For this review, take the finished solid that the model builds, in its own axes (mm). Face numbers are marked on the shaded views. A direction names the side the tool comes from. Coordinates: 2 decimals unless noted, no trailing zeros. Order: outer loops, then holes, each group sorted by start corner. A loop starts at its lowest first (then second) coordinate and runs counter-clockwise, first axis right, second up. Notation, with made-up numbers: (59.5, 19.25) -> (77.5, 19.25) arc R23 cw to (77.5, 35.25) -> close; hole circle Ø9 at (0.25, 58.25). An arc over 180 degrees is marked (long way). Answer as a JSON object with one key per item and string values. Group by question number.
1) Add section A-A, the plane y = -1. Count the separate pieces of the cut face and the enclosed holes in it, then the cut area to 3 significant figures.
2) Add section D-D, the plane y = 27. Write out the cut boundary in (x, z).
3) Machinability: for the marked faces 1, 2 and 3, which of the approach directions +Z, -Z, +X, -X, +Y, -Y give a long, thin tool a straight path to every point of the face, cutting with its end or side? Answer none if there is none.
4) Add section C-C, the plane x = 15.5. Write out the cut boundary in (y, z), then the cut area to 3 significant figures.
5) Draft analysis for pull direction Y (two halves, no side actions). For the marked faces 4, 5 and 6, state which applies: +Y half, -Y half, draft (parallel to the pull), parting line (faces both ways), or undercut.
6) For pin 1 (6 mm diameter, centred on x = -12.5, y = 18, fed in from -Z); pin 2 (5 mm diameter, centred on y = 16.5, z = 11, fed in from +X); pin 3 (3.5 mm diameter, centred on x = 7.5, y = 28.42, fed in from -Z); pin 4 (17.5 mm diameter, centred on x = -35, y = -1, fed in from +Z), all flat-tipped, find the tip position at first contact; note any pin that passes through.
7) Add section B-B, the plane x = -17.5. Write out the cut boundary in (y, z).
8) Wall thickness on L1, parallel to Y at x = 7.5, z = 14.1; L2, parallel to X at y = 0, z = 12.75; L3, parallel to Y at x = -9, z = 5.75: over which ranges is each line inside the solid? List them lowest first.
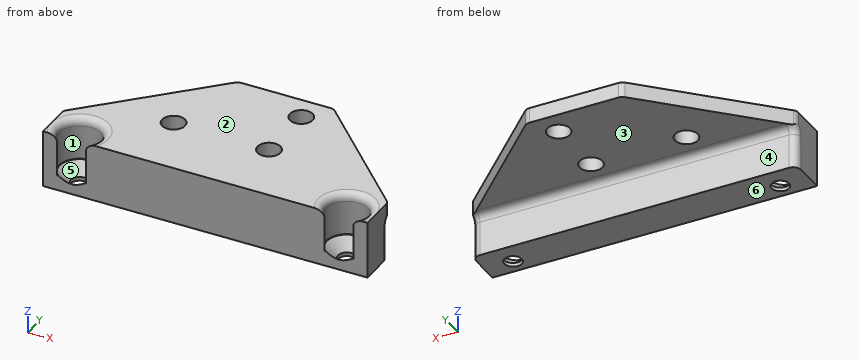
from build123d import *

# Parameters (mm, degrees)
SKETCH1_W           = 85
SKETCH1_H           = 10
BOSS_EXTRUDE1_DEPTH = 15
SKETCH3_R           = 2.292918
CUT_EXTRUDE1_DEPTH  = 100
LPATTERN1_COUNT     = 2
LPATTERN1_PITCH     = 70
SKETCH7_W           = 85
SKETCH7_H           = 4
BOSS_EXTRUDE5_DEPTH = 30
SKETCH8_R           = 3
CUT_EXTRUDE2_DEPTH  = 25
LPATTERN2_START     = 11
LPATTERN2_OUTLINE_R = 3
LPATTERN2_DEPTH     = 4
CHAMFER2_SIZE       = 30
FILLET3_START       = -1
FILLET3_DEPTH       = 10
FILLET3_START_2     = 1.5411
FILLET3_2_DEPTH     = 14.4589
FILLET3_START_3     = 9
FILLET3_3_DEPTH     = 2.164784
FILLET3_5_DEPTH     = 2
FILLET3_START_4     = 11
FILLET3_6_OUTLINE_R = 3
FILLET3_6_DEPTH     = 0.164784
SKETCH9_R           = 5.5
CUT_EXTRUDE7_DEPTH  = 11
LPATTERN3_COUNT     = 2
LPATTERN3_PITCH     = 70
CHAMFER3_SIZE       = 3
FILLET4_R           = 2


with BuildPart() as part:
    # Sketch1 → Boss-Extrude1 (new body)
    with BuildSketch(Plane.XY):
        Rectangle(SKETCH1_W, SKETCH1_H)
    extrude(amount=BOSS_EXTRUDE1_DEPTH)

    # Sketch3 → Cut-Extrude1 (cut)
    with BuildSketch(Plane.XY.offset(15)):
        with Locations((-35, -1)):
            Circle(SKETCH3_R)
    cut_extrude1 = extrude(amount=-CUT_EXTRUDE1_DEPTH, mode=Mode.SUBTRACT)

    # LPattern1: Cut-Extrude1 ×2
    with Locations(*[(i * LPATTERN1_PITCH, 0, 0) for i in range(1, LPATTERN1_COUNT)]):
        add(cut_extrude1, mode=Mode.SUBTRACT)

    # Sketch7 → Boss-Extrude5 (add)
    with BuildSketch(Plane(origin=(0, 5, 0), x_dir=(1, 0, 0), z_dir=(0, 1, 0))):
        with Locations((0, -13)):
            Rectangle(SKETCH7_W, SKETCH7_H)
    extrude(amount=BOSS_EXTRUDE5_DEPTH)

    # Sketch8 → Cut-Extrude2 (cut)
    with BuildSketch(Plane.XY.offset(15)):
        with Locations((7.5, 12.421962)):
            Circle(SKETCH8_R)
    extrude(amount=-CUT_EXTRUDE2_DEPTH, mode=Mode.SUBTRACT)

    # LPattern2: read off the stored shape, not the designer's step
    # LPattern2 outline → LPattern2 (cut)
    with BuildSketch(Plane.XY.offset(LPATTERN2_START)):
        with Locations((-17.5, 12.421962)):
            Circle(LPATTERN2_OUTLINE_R)
        with Locations((7.5, 28.421962)):
            Circle(LPATTERN2_OUTLINE_R)
    extrude(amount=LPATTERN2_DEPTH, mode=Mode.SUBTRACT)

    # Chamfer2
    chamfer2_edges = [part.edges().sort_by_distance(p)[0] for p in [
        (42.5, 35, 13),
        (-42.5, 35, 13),
    ]]
    chamfer(chamfer2_edges, length=CHAMFER2_SIZE)

    # Fillet3: read off the stored shape, not the designer's step
    # Fillet3 outline → Fillet3 (cut)
    with BuildSketch(Plane.XY.offset(FILLET3_START)):
        with BuildLine():
            ThreePointArc((40.5, 5), (41.914214, 4.414214), (42.5, 3))
            Line((42.5, 3), (42.5, 5))
            Line((42.5, 5), (40.5, 5))
        make_face()
        with BuildLine():
            ThreePointArc((-42.5, 3), (-41.914214, 4.414214), (-40.5, 5))
            Line((-40.5, 5), (-42.5, 5))
            Line((-42.5, 5), (-42.5, 3))
        make_face()
    extrude(amount=FILLET3_DEPTH, mode=Mode.SUBTRACT)

    # Fillet3 2 outline → Fillet3 2 (cut)
    with BuildSketch(Plane.XY.offset(FILLET3_START_2)):
        with BuildLine():
            Line((42.5, 4.171573), (42.5, 5))
            Line((42.5, 5), (41.914214, 5.585786))
            ThreePointArc((41.914214, 5.585786), (42.347759, 4.93694), (42.5, 4.171573))
        make_face()
        with BuildLine():
            Line((-41.914214, 5.585786), (-42.5, 5))
            Line((-42.5, 5), (-42.5, 4.171573))
            ThreePointArc((-42.5, 4.171573), (-42.347759, 4.93694), (-41.914214, 5.585786))
        make_face()
        with BuildLine():
            ThreePointArc((11.671573, 35), (12.43694, 34.847759), (13.085786, 34.414214))
            Line((13.085786, 34.414214), (12.5, 35))
            Line((12.5, 35), (11.671573, 35))
        make_face()
        with BuildLine():
            Line((-12.5, 35), (-13.085786, 34.414214))
            ThreePointArc((-13.085786, 34.414214), (-12.43694, 34.847759), (-11.671573, 35))
            Line((-11.671573, 35), (-12.5, 35))
        make_face()
    extrude(amount=FILLET3_2_DEPTH, mode=Mode.SUBTRACT)

    # Fillet3 3 outline → Fillet3 3 (add)
    with BuildSketch(Plane.XY.offset(FILLET3_START_3)):
        with BuildLine():
            Line((-42.320359, 5), (42.320359, 5))
            ThreePointArc((42.320359, 5), (42.143594, 5.311133), (41.914214, 5.585786))
            Line((41.914214, 5.585786), (13.085786, 34.414214))
            ThreePointArc((13.085786, 34.414214), (12.43694, 34.847759), (11.671573, 35))
            Line((11.671573, 35), (-11.671573, 35))
            ThreePointArc((-11.671573, 35), (-12.43694, 34.847759), (-13.085786, 34.414214))
            Line((-13.085786, 34.414214), (-41.914214, 5.585786))
            ThreePointArc((-41.914214, 5.585786), (-42.143594, 5.311133), (-42.320359, 5))
        make_face()
    extrude(amount=FILLET3_3_DEPTH)

    # Fillet3 4 outline → Fillet3 4 (revolve, cut)
    with BuildSketch(Plane(origin=(0, 7, 9), x_dir=(0, 1, 0), z_dir=(0, 0, -1))):
        with BuildLine():
            Line((4, 42.5), (0, 42.5))
            Line((0, 42.5), (0, -42.5))
            Line((0, -42.5), (4, -42.5))
            ThreePointArc((4, -42.5), (2.585786, -41.914214), (2, -40.5))
            Line((2, -40.5), (2, 40.5))
            ThreePointArc((2, 40.5), (2.585786, 41.914214), (4, 42.5))
        make_face()
    revolve(axis=Axis((0, 7, 9), (1, 0, 0)), mode=Mode.SUBTRACT)

    # Fillet3 5 outline → Fillet3 5 (cut)
    with BuildSketch(Plane.XY.offset(FILLET3_START_3)):
        with BuildLine():
            Line((11.671573, 35), (-11.671573, 35))
            ThreePointArc((-11.671573, 35), (-12.43694, 34.847759), (-13.085786, 34.414214))
            Line((-13.085786, 34.414214), (-40.5, 7))
            Line((-40.5, 7), (40.5, 7))
            Line((40.5, 7), (13.085786, 34.414214))
            ThreePointArc((13.085786, 34.414214), (12.43694, 34.847759), (11.671573, 35))
        make_face()
    extrude(amount=FILLET3_5_DEPTH, mode=Mode.SUBTRACT)

    # Fillet3 6 outline → Fillet3 6 (cut)
    with BuildSketch(Plane.XY.offset(FILLET3_START_4)):
        with Locations((7.5, 28.421962)):
            Circle(FILLET3_6_OUTLINE_R)
        with Locations((7.5, 12.421962)):
            Circle(FILLET3_6_OUTLINE_R)
        with Locations((-17.5, 12.421962)):
            Circle(FILLET3_6_OUTLINE_R)
    extrude(amount=FILLET3_6_DEPTH, mode=Mode.SUBTRACT)

    # Sketch9 → Cut-Extrude7 (cut)
    with BuildSketch(Plane.XY.offset(15)):
        with Locations((-35, -1)):
            Circle(SKETCH9_R)
    cut_extrude7 = extrude(amount=-CUT_EXTRUDE7_DEPTH, mode=Mode.SUBTRACT)

    # LPattern3: Cut-Extrude7 ×2
    with Locations(*[(i * LPATTERN3_PITCH, 0, 0) for i in range(1, LPATTERN3_COUNT)]):
        add(cut_extrude7, mode=Mode.SUBTRACT)

    # Chamfer3
    # the kernel refuses this chamfer: 3 mm, written as the material it takes off along each edge
    with BuildSketch(Plane(origin=(-35, -1, 4), x_dir=(1, 0, 0), z_dir=(0, -1, 0))) as chamfer3_piece_1:
        Polygon((2.292918 + CHAMFER3_SIZE, 0), (2.292918, -CHAMFER3_SIZE), (2.292918, 0), align=None)
    revolve(axis=Axis((-35, -1, 4), (0, 0, 1)), mode=Mode.SUBTRACT)
    with BuildSketch(Plane(origin=(35, -1, 4), x_dir=(1, 0, 0), z_dir=(0, -1, 0))) as chamfer3_piece_2:
        Polygon((2.292918 + CHAMFER3_SIZE, 0), (2.292918, -CHAMFER3_SIZE), (2.292918, 0), align=None)
    revolve(axis=Axis((35, -1, 4), (0, 0, 1)), mode=Mode.SUBTRACT)

    # Fillet4
    fillet4_edges = [part.edges().sort_by_distance(p)[0] for p in [
        (-35, 4.5, 15),
        (35, 4.5, 15),
    ]]
    fillet(fillet4_edges, radius=FILLET4_R - 0.0001)  # a hair under: the kernel refuses the full size


solid = part.part
Output values:
{
 "1": {"separate pieces": "3", "enclosed holes": "0", "area": "975 mm²"},
 "2": {"outline": "(-20.5, 11) -> (4.86, 11) -> (4.86, 15) -> (-20.5, 15) -> close; (10.14, 11) -> (20.5, 11) -> (20.5, 15) -> (10.14, 15) -> close"},
 "3": {"face 1": "+Z", "face 2": "+Z, +X, -X, +Y, -Y", "face 3": "-Z, +X, -X, +Y"},
 "4": {"outline": "(-5, 0) -> (5, 0) -> (5, 9) arc R2 cw to (7, 11) -> (32, 11) -> (32, 15) -> (-5, 15) -> close", "area": "259 mm²"},
 "5": {"face 4": "+Y half", "face 5": "undercut", "face 6": "draft"},
 "6": {"pin 1": "stops at z = 11", "pin 2": "stops at x = 33.5", "pin 3": "passes through", "pin 4": "stops at z = 15"},
 "7": {"outline": "(-5, 0) -> (5, 0) -> (5, 9) arc R2 cw to (7, 11) -> (9.42, 11) -> (9.42, 15) -> (-5, 15) -> close; (15.42, 11) -> (30, 11) -> (30, 15) -> (15.42, 15) -> close"},
 "8": {"L1": "y = -5 to 9.42, 15.42 to 25.42, 31.42 to 35", "L2": "x = -42.5 to -40.41, -29.59 to 29.59, 40.41 to 42.5", "L3": "y = -5 to 5"}
}
